from build123d import *

# Parameters (mm, degrees)
SKETCH1_R           = 2.5
SKETCH1_R_2         = 2.6
BOSS_EXTRUDE1_DEPTH = 6
BOSS_EXTRUDE2_DEPTH = 3
CHAMFER1_SIZE       = 2


with BuildPart() as part:
    # Sketch1 → Boss-Extrude1 (new body)
    with BuildSketch(Plane.XY):
        Polygon((2998.461039771, 1261.470901479), (2998.461039771, 1206.670901479), (2962.016271034, 1185.629504438), (2914.558078907, 1213.029504438), (2914.558078907, 1255.11229852), (2962.016271034, 1282.51229852), align=None)
        with Locations((2990.961039771, 1221.070901479)):
            Circle(SKETCH1_R, mode=Mode.SUBTRACT)
        with Locations((2980.961039771, 1234.070901479)):
            Circle(SKETCH1_R, mode=Mode.SUBTRACT)
        with Locations((2990.961039771, 1247.070901479)):
            Circle(SKETCH1_R, mode=Mode.SUBTRACT)
        with Locations((2953.699650408, 1269.050441325)):
            Circle(SKETCH1_R, mode=Mode.SUBTRACT)
        with Locations((2930.374699533, 1255.583774658)):
            Circle(SKETCH1_R_2, mode=Mode.SUBTRACT)
        with Locations((2947.03717497, 1214.484949004)):
            Circle(SKETCH1_R, mode=Mode.SUBTRACT)
        with Locations((2953.699650408, 1199.091361633)):
            Circle(SKETCH1_R, mode=Mode.SUBTRACT)
        with Locations((2930.374699533, 1212.5580283)):
            Circle(SKETCH1_R_2, mode=Mode.SUBTRACT)
        with Locations((2947.03717497, 1253.656853954)):
            Circle(SKETCH1_R_2, mode=Mode.SUBTRACT)
    extrude(amount=BOSS_EXTRUDE1_DEPTH)

    # Sketch2 → Boss-Extrude2 (add)
    with BuildSketch(Plane.XY.offset(6)):
        Polygon((2916.290129714, 1212.029504438), (2928.790129714, 1233.680139532), (2972.784220226, 1208.280139532), (2960.284220226, 1186.629504438), (2962.016271034, 1185.629504438), (2998.461039771, 1206.670901479), (2998.461039771, 1208.670901479), (2973.461039771, 1208.670901479), (2973.461039771, 1259.470901479), (2998.461039771, 1259.470901479), (2998.461039771, 1261.470901479), (2962.016271034, 1282.51229852), (2960.284220226, 1281.51229852), (2972.784220226, 1259.861663425), (2928.790129714, 1234.461663425), (2916.290129714, 1256.11229852), (2914.558078907, 1255.11229852), (2914.558078907, 1213.029504438), align=None)
    extrude(amount=BOSS_EXTRUDE2_DEPTH)

    # Chamfer1
    chamfer1_edges = [part.edges().sort_by_distance(p)[0] for p in [
        (2980.238655403, 1196.150202958, 0),
        (2938.28717497, 1199.329504438, 0),
        (2914.558078907, 1234.070901479, 0),
        (2938.28717497, 1268.81229852, 0),
        (2980.238655403, 1271.991599999, 0),
        (2998.461039771, 1234.070901479, 0),
    ]]
    chamfer(chamfer1_edges, length=CHAMFER1_SIZE)


solid = part.part
Here's how the part is built. I have some questions about the finished solid (model axes, mm). A direction names the side the tool comes from. Coordinates: 2 decimals unless noted, no trailing zeros. Order: outer loops, then holes, each group sorted by start corner. A loop starts at its lowest first (then second) coordinate and runs counter-clockwise, first axis right, second up. Notation, with made-up numbers: M 2.25,-29 L 42.25,-29 A21 cw 42.25,-10 Z; hole C -26.5,79 d2. An arc over 180 degrees is marked long. Answer as CSV lines item,"result". Start each with the question number.
1. I want a section at A-A, the plane z = 4.75. Count the separate pieces of the cut face and the enclosed holes in it, and give its area (3 significant figures).
2. I want a section at B-B, the plane x = 2968. Write out the boundary of the cut face in (y, z), and give its area (3 significant figures).
3. On a 3-axis mill with a long thin cutter (end or side, diameter ignored), from which of +Z, -Z, +X, -X, +Y, -Y can I reach the whole of each face in a straight line? I mean faces 5 (the cylindrical face through (2954.9, 1196.9, 3)), 6 (the flat face through (2966.447, 1270.839, 7.479)), 7 (the flat face through (2979.49, 1271.28, 1.01)), 8 (the flat face through (2945, 1210, 6)), 9 (the flat face through (2986, 1208.671, 7)). Say none if no direction works.
4. For pin 1 (3 mm diameter, centred on x = 2937.5, z = 4, fed in from +Y); pin 2 (0.9 mm diameter, centred on x = 2989, z = 8, fed in from -Y); pin 3 (6 mm diameter, centred on x = 2990.96, y = 1247.07, fed in from +Z); pin 4 (4.5 mm diameter, centred on x = 2953.7, y = 1269.05, fed in from +Z), each with a flat end and sliding along its axis, tell me the tip position at first contact or that it passes through.
5. I want a section at C-C, the plane y = 1238.5. Write out the boundary of the cut face in (x, z).
6. We'd pull the mould along X, two halves only. Please class faces 1 (the cylindrical face through (2949.517, 1254.438, 2.958)), 2 (the flat face through (2915.57, 1233.78, 0.99)), 3 (the cylindrical face through (2932.776, 1254.588, 2.958)), 4 (the flat face through (2957, 1235, 0)): released by +X, released by -X, zero draft, split by the parting line, or undercut.
7. I need wall thicknesses on line 1 (Y direction, x = 2931, z = 1.5); line 2 (Z direction, x = 2983.5, y = 1237.5); line 3 (X direction, y = 1236.5, z = 6.75). Which ranges of each line are inside material? Lowest first, please. Write a range as [from, to].
8. I want a section at D-D, the plane y = 1275. Write out the boundary of the cut face in (x, z).
Recorded:
1,separate pieces,"1"
1,enclosed holes,"9"
1,area,"5,880 mm2"
2,outline,"M 1189.08,2 L 1191.39,0 L 1276.75,0 L 1279.06,2 L 1279.06,9 L 1268.15,9 L 1268.15,6 L 1257.1,6 L 1257.1,9 L 1211.04,9 L 1211.04,6 L 1199.99,6 L 1199.99,9 L 1189.08,9 Z"
2,area,"739 mm2"
3,face 5,"+Z, -Z"
3,face 6,"+Z, -X"
3,face 7,"-Z, +X, +Y"
3,face 8,"+Z"
3,face 9,"+Z, +X"
4,pin 1,"stops at y = 1269.22"
4,pin 2,"stops at y = 1200.95"
4,pin 3,"stops at z = 6"
4,pin 4,"passes through"
5,outline,"M 2914.56,2 L 2916.56,0 L 2996.46,0 L 2998.46,2 L 2998.46,6 L 2973.46,6 L 2973.46,9 L 2935.78,9 L 2935.78,6 L 2926.46,6 L 2926.46,9 L 2914.56,9 Z"
6,face 1,"undercut"
6,face 2,"released by -X"
6,face 3,"undercut"
6,face 4,"zero draft"
7,line 1,"y = [1204.11, 1210.03], [1215.08, 1253.06], [1258.11, 1264.03]"
7,line 2,"z = [0, 6]"
7,line 3,"x = [2914.56, 2927.61], [2932.32, 2973.46]"
8,outline,"M 2949,2 L 2953,0 L 2971.03,0 L 2975.03,2 L 2975.03,9 L 2964.04,9 L 2964.04,6 L 2949,6 Z"
